from build123d import *

# Parameters (mm, degrees)
F0_R     = 1.2573
F1_DEPTH = 3.175


with BuildPart() as f1:
    # F0 (on Top) → F1 (new body)
    with BuildSketch(Plane.XY):
        with BuildLine():
            Line((-104.775, 133.35), (-104.775, 101.6))
            Line((-104.775, 101.6), (-111.823455, 108.648455))
            ThreePointArc((-111.823455, 108.648455), (-113.601545, 108.648455), (-113.601545, 110.426545))
            Line((-113.601545, 110.426545), (-120.65, 117.475))
            Line((-120.65, 117.475), (-127.698455, 124.523455))
            ThreePointArc((-127.698455, 124.523455), (-129.476545, 124.523455), (-129.476545, 126.301545))
            Line((-129.476545, 126.301545), (-136.525, 133.35))
            Line((-136.525, 133.35), (-136.525, 101.6))
            Line((-136.525, 101.6), (-133.35, 101.6))
            Line((-133.35, 101.6), (-133.35, 60.325))
            Line((-133.35, 60.325), (-133.35, 50.8))
            Line((-133.35, 50.8), (-133.35, -50.8))
            Line((-133.35, -50.8), (-133.35, -60.325))
            Line((-133.35, -60.325), (-133.35, -101.6))
            Line((-133.35, -101.6), (-136.525, -101.6))
            Line((-136.525, -101.6), (-136.525, -133.35))
            Line((-136.525, -133.35), (-60.325, -133.35))
            Line((-60.325, -133.35), (-50.8, -133.35))
            Line((-50.8, -133.35), (50.8, -133.35))
            Line((50.8, -133.35), (60.325, -133.35))
            Line((60.325, -133.35), (136.525, -133.35))
            Line((136.525, -133.35), (136.525, -101.6))
            Line((136.525, -101.6), (133.35, -101.6))
            Line((133.35, -101.6), (133.35, -60.325))
            Line((133.35, -60.325), (133.35, -50.8))
            Line((133.35, -50.8), (133.35, 0))
            Line((133.35, 0), (133.35, 50.8))
            Line((133.35, 50.8), (133.35, 60.325))
            Line((133.35, 60.325), (133.35, 101.6))
            Line((133.35, 101.6), (136.525, 101.6))
            Line((136.525, 101.6), (136.525, 133.35))
            Line((136.525, 133.35), (104.775, 133.35))
            Line((104.775, 133.35), (101.6, 133.35))
            Line((101.6, 133.35), (60.325, 133.35))
            Line((60.325, 133.35), (50.8, 133.35))
            Line((50.8, 133.35), (0, 133.35))
            Line((0, 133.35), (-50.8, 133.35))
            Line((-50.8, 133.35), (-60.325, 133.35))
            Line((-60.325, 133.35), (-101.6, 133.35))
            Line((-101.6, 133.35), (-104.775, 133.35))
        make_face()
        with Locations((-128.5875, -125.4125)):
            Circle(F0_R, mode=Mode.SUBTRACT)
        with Locations((-112.7125, -109.5375)):
            Circle(F0_R, mode=Mode.SUBTRACT)
        with Locations((112.7125, -109.5375)):
            Circle(F0_R, mode=Mode.SUBTRACT)
        with Locations((128.5875, -125.4125)):
            Circle(F0_R, mode=Mode.SUBTRACT)
        Polygon((0, 101.6), (101.6, 101.6), (101.6, 0), (101.6, -101.6), (0, -101.6), (-101.6, -101.6), (-101.6, 0), (-101.6, 101.6), align=None, mode=Mode.SUBTRACT)
        with Locations((112.7125, 109.5375)):
            Circle(F0_R, mode=Mode.SUBTRACT)
        with Locations((128.5875, 125.4125)):
            Circle(F0_R, mode=Mode.SUBTRACT)
        with BuildLine():
            Line((-111.823455, 108.648455), (-104.775, 101.6))
            Line((-104.775, 101.6), (-104.775, 133.35))
            Line((-104.775, 133.35), (-136.525, 133.35))
            Line((-136.525, 133.35), (-129.476545, 126.301545))
            ThreePointArc((-129.476545, 126.301545), (-128.106352, 126.574094), (-127.3302, 125.4125))
            ThreePointArc((-127.3302, 125.4125), (-127.425906, 124.931352), (-127.698455, 124.523455))
            Line((-127.698455, 124.523455), (-120.65, 117.475))
            Line((-120.65, 117.475), (-113.601545, 110.426545))
            ThreePointArc((-113.601545, 110.426545), (-112.231352, 110.699094), (-111.4552, 109.5375))
            ThreePointArc((-111.4552, 109.5375), (-111.550906, 109.056352), (-111.823455, 108.648455))
        make_face()
        Polygon((-60.325, 168.275), (-60.325, 133.35), (-50.8, 133.35), (-50.8, 158.75), (0, 158.75), (50.8, 158.75), (50.8, 133.35), (60.325, 133.35), (60.325, 168.275), (0, 168.275), align=None)
        Polygon((-133.35, 50.8), (-133.35, 60.325), (-168.275, 60.325), (-168.275, 0), (-168.275, -60.325), (-133.35, -60.325), (-133.35, -50.8), (-158.75, -50.8), (-158.75, 0), (-158.75, 50.8), align=None)
        Polygon((-50.8, -133.35), (-60.325, -133.35), (-60.325, -168.275), (0, -168.275), (60.325, -168.275), (60.325, -133.35), (50.8, -133.35), (50.8, -158.75), (0, -158.75), (-50.8, -158.75), align=None)
        Polygon((168.275, 60.325), (133.35, 60.325), (133.35, 50.8), (158.75, 50.8), (158.75, 0), (158.75, -50.8), (133.35, -50.8), (133.35, -60.325), (168.275, -60.325), (168.275, 0), align=None)
    extrude(amount=F1_DEPTH)


solid = f1.part
Geometry: final body of the model. Coordinates: model frame, mm. Coordinates: 2 decimals unless noted, no trailing zeros. Order: outer loops, then holes, each group sorted by start corner. A loop starts at its lowest first (then second) coordinate and runs counter-clockwise, first axis right, second up.
(1) First-contact query: pin 1 (1.5 mm diameter, centred on x = -128, z = 0.5, fed in from -Y); pin 2 (1.6 mm diameter, centred on x = 144, z = 1, fed in from +Y) (3 decimals); pin 3 (4 mm diameter, centred on x = 128.59, y = -125.41, fed in from -Z); pin 4 (1 mm diameter, centred on y = -82, z = 1.5, fed in from +X). Flat tips, straight axial feed; report the tip coordinate or a pass-through.
(2) Section query D-D (x = -93). Return the cut outline in (y, z) (3 decimals), plus the area to 3 significant figures.
(3) Material intervals for probe 1 along X at (y, z) = (-50.5, 2) (3 decimals); probe 2 along X at (y, z) = (-125, 1.3) (3 decimals), sorted ascending.
(4) Section query A-A (x = 18). Return the cut outline in (y, z) (3 decimals).
(5) Section query C-C (x = 146). Return the cut outline in (y, z) (3 decimals).
Solution:
1. pin 1: stops at y = -133.35
1. pin 2: stops at y = 60.325
1. pin 3: stops at z = 0
1. pin 4: stops at x = 133.35
2. outline: (-133.35, 0) - (-101.6, 0) - (-101.6, 3.175) - (-133.35, 3.175) - close; (101.6, 0) - (133.35, 0) - (133.35, 3.175) - (101.6, 3.175) - close
2. area: 202 mm2
3. probe 1: x = -168.275 to -158.75, -133.35 to -101.6, 101.6 to 133.35, 158.75 to 168.275
3. probe 2: x = -136.525 to -129.775, -127.4 to 127.4, 129.775 to 136.525
4. outline: (-168.275, 0) - (-158.75, 0) - (-158.75, 3.175) - (-168.275, 3.175) - close; (-133.35, 0) - (-101.6, 0) - (-101.6, 3.175) - (-133.35, 3.175) - close; (101.6, 0) - (133.35, 0) - (133.35, 3.175) - (101.6, 3.175) - close; (158.75, 0) - (168.275, 0) - (168.275, 3.175) - (158.75, 3.175) - close
5. outline: (-60.325, 0) - (-50.8, 0) - (-50.8, 3.175) - (-60.325, 3.175) - close; (50.8, 0) - (60.325, 0) - (60.325, 3.175) - (50.8, 3.175) - close
